Could you check a few things on this drawing? It's one solid part, dimensions in mm from its lowest x, y, z. A direction names the side the tool comes from. Give positions to 0.01 mm unless a question says otherwise; leave off trailing zeros. Loops run counter-clockwise (first coordinate to the right, second up) from the corner with the lowest first, then second, coordinate; pieces in that order, holes last. Notation, with made-up numbers: (85.5, -19) - (98.5, -19) arc R28 ccw to (98.5, 2) - close; hole circle Ø10 at (57.25, 70.25). An arc over 180 degrees is marked (long way). Answer as a JSON object with one key per item and string values.
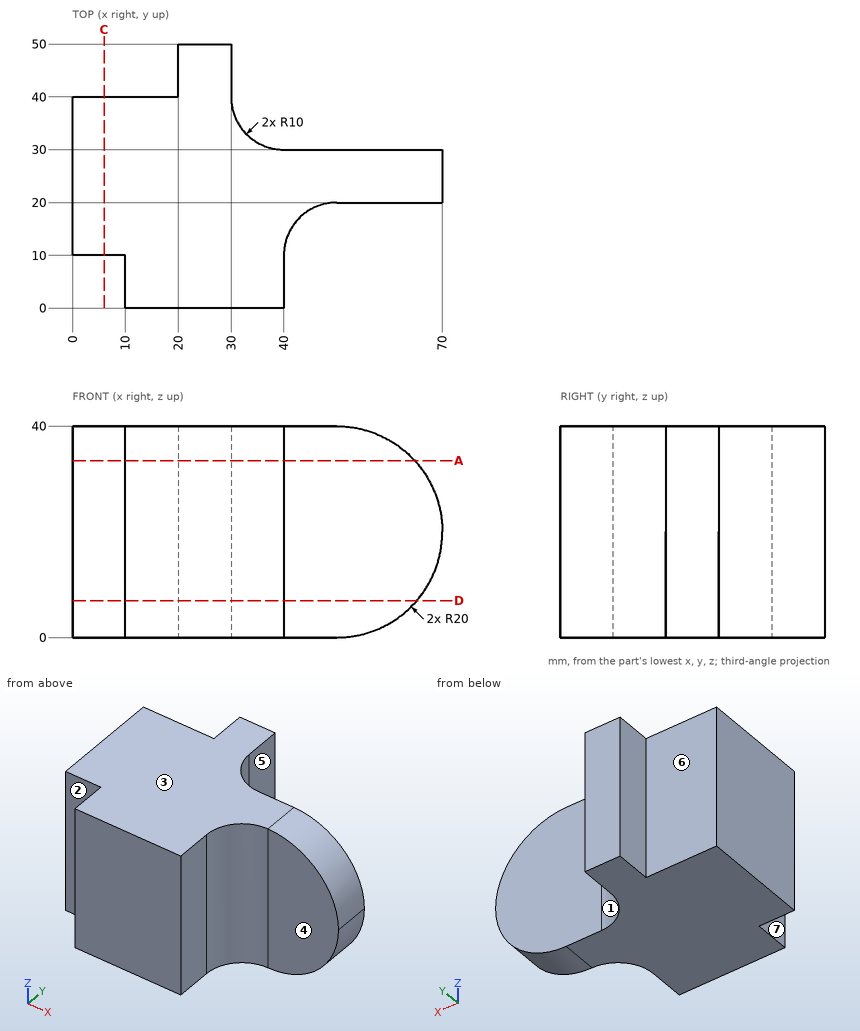
1) Imagine slicing it at C-C on x = 6. Write out the boundary of the cut face in (y, z), and give its area (3 significant figures).
Check sheet entries:
{"outline": "(10, 0) - (40, 0) - (40, 40) - (10, 40) - close", "area": "1,200 mm2"}
2) Imagine slicing it at A-A on z = 33.5. Write out the boundary of the cut face in (x, y), and give its area (3 significant figures).
Check sheet entries:
{"outline": "(0, 10) - (10, 10) - (10, 0) - (40, 0) - (40, 10) arc R10 cw to (50, 20) - (64.76, 20) - (64.76, 30) - (40, 30) arc R10 cw to (30, 40) - (30, 50) - (20, 50) - (20, 40) - (0, 40) - close", "area": "1,790 mm2"}
3) If we mould it in two halves opening along Y, with no side actions, what happens to the marked faces 1, 2 and 3? For each: released by +Y, released by -Y, zero draft, split by the parting line, or undercut.
Check sheet entries:
{"face 1": "released by +Y", "face 2": "released by -Y", "face 3": "zero draft"}
4) I'm going to push flat-ended pins straight in: P1, Ø8, axis at y = 4.5, z = 23.5, coming from the +X side; P2, Ø6, axis at x = 42, z = 25.5, coming from the +Y side; P3, Ø5, axis at y = 21.5, z = 16, coming from the +X side; P4, Ø8, axis at y = 42.5, z = 12.5, coming from the -X side. Where does each tip first touch, or does it pass through?
Check sheet entries:
{"P1": "x = 40", "P2": "y = 30.05", "P3": "x = 69.94", "P4": "x = 0"}
5) Imagine slicing it at D-D on z = 7. Write out the boundary of the cut face in (x, y), and give its area (3 significant figures).
Check sheet entries:
{"outline": "(0, 10) - (10, 10) - (10, 0) - (40, 0) - (40, 10) arc R10 cw to (50, 20) - (65.2, 20) - (65.2, 30) - (40, 30) arc R10 cw to (30, 40) - (30, 50) - (20, 50) - (20, 40) - (0, 40) - close", "area": "1,790 mm2"}
6) Which directions (+Z, -Z, +X, -X, +Y, -Y) give clear straight access to the entire face, cutting with the end or side of a thin tool? Please do the marked faces 4, 5, 6 and 7.
Check sheet entries:
{"face 4": "+Z, -Z, +X, -Y", "face 5": "+Z, -Z, +X, +Y", "face 6": "+Z, -Z, -X, +Y", "face 7": "+Z, -Z, -X, -Y"}
7) I need wall thicknesses on L1, parallel to Y at x = 61.5, z = 31.5; L2, parallel to X at y = 9, z = 17. Which ranges of each line are inside material? Lowest first, please.
Check sheet entries:
{"L1": "20 to 30", "L2": "10 to 40"}
